Check sheet for the drawn part. Datum: minimum x, y, z corner. Units: mm. A direction names the side the tool comes from. Round coordinates to 2 decimals unless told otherwise and drop trailing zeros. Order: outer loops, then holes, each group sorted by start corner. A loop starts at its lowest first (then second) coordinate and runs counter-clockwise, first axis right, second up. Notation, with made-up numbers: M 11.25,-20 L 67.25,-20 A24 ccw 67.25,0 Z; hole C 27.5,7.5 d3. An arc over 180 degrees is marked long. Use one line per item in the form item = value. Start each with the question number.
Item 1: Cross-section at D-D on z = 17.5. Enter the section's corners in (x, y).
Item 2: Go/stop test with flat-tipped pins: pin 1 Ø1 at (x, y) = (26, 13.5) entering from -Z; pin 2 Ø11 at (x, z) = (9, 11.5) entering from +Y; pin 3 Ø15 at (x, y) = (21, 14) entering from +Z. Record where each tip stops, or that it passes through.
Item 3: Tool access check on the marked faces 5, 6, 7 and 8. Record the directions out of +Z, -Z, +X, -X, +Y, -Y that give a thin tool (end or side, any length) a straight path to the whole face; none if there is none.
Item 4: Cross-section at A-A on z = 10. Enter the section's corners in (x, y).
Item 5: Cross-section at B-B on x = 15. Enter the section's corners in (y, z).
Item 6: Release check for a two-part mould opening along Z. For the marked faces 1, 2, 3 and 4 record: +Z half, -Z half, draft (parallel to the pull), parting line (faces both ways), or undercut.
Item 7: Thickness scan on probe 1 along X at (y, z) = (16, 10); probe 2 along Z at (x, y) = (24, 19.75); probe 3 along Z at (x, y) = (8, 22.75). Record the ranges inside material, lowest first. Write a range as [from, to].
Item 8: Cross-section at C-C on y = 19. Enter the section's corners in (x, z).
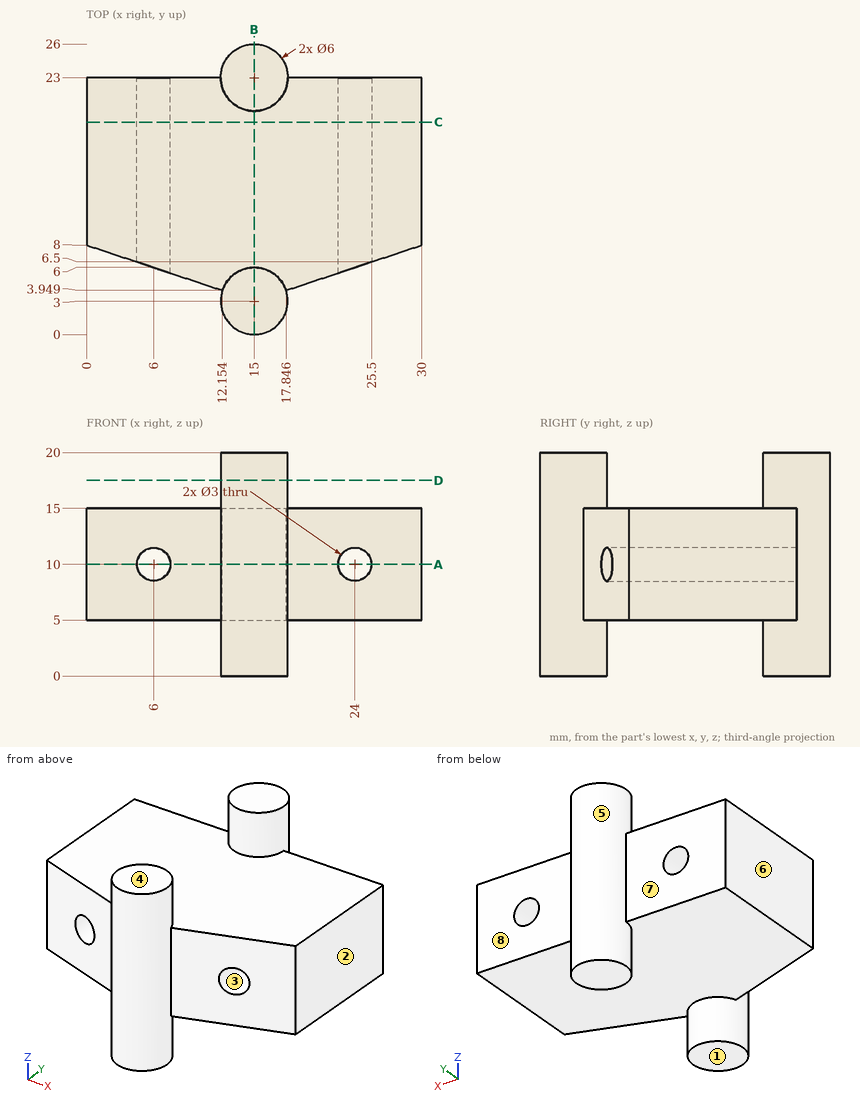
Output values:
q1.outline = C 15,3 d6; C 15,23 d6
q2.pin_1 = 5
q2.pin_2 = 25.96
q2.pin_3 = 15
q3.face_5 = none
q3.face_6 = +Z, -Z, -X, +Y, -Y
q3.face_7 = +Z, -Z, -X, +Y
q3.face_8 = +Z, -Z, +X, +Y
q4.outline = M 0,8 L 4.5,6.5 L 4.5,23 L 0,23 Z; M 7.5,5.5 L 12.15,3.95 A3 ccw long 17.85,3.95 L 22.5,5.5 L 22.5,23 L 18,23 A3 ccw 12,23 L 7.5,23 Z; M 25.5,6.5 L 30,8 L 30,23 L 25.5,23 Z
q5.outline = M 0,0 L 6,0 L 6,5 L 20,5 L 20,0 L 26,0 L 26,20 L 20,20 L 20,15 L 6,15 L 6,20 L 0,20 Z
q6.face_1 = -Z half
q6.face_2 = draft
q6.face_3 = undercut
q6.face_4 = +Z half
q7.probe_1 = [0, 4.5], [7.5, 22.5], [25.5, 30]
q7.probe_2 = [5, 8.5], [11.5, 15]
q7.probe_3 = [5, 15]
q8.outline = M 0,5 L 30,5 L 30,15 L 0,15 Z; hole C 6,10 d3; hole C 24,10 d3
